from build123d import *

# Parameters (mm, degrees)
SKIZZE1_R                            = 6.1
AUFSATZ_LINEAR_AUSTRAGEN1_DEPTH      = 6
SCHNITT_LINEAR_AUSTRAGEN1_REACH      = 48.187
SCHNITT_LINEAR_AUSTRAGEN1_END_RADIUS = 6.1
SKIZZE2_R                            = 2.2
VERRUNDUNG1_R                        = 6
FASE1_SIZE                           = 0.5


with BuildPart() as part:
    # Skizze1 → Aufsatz-Linear austragen1 (new body)
    with BuildSketch(Plane.XY):
        with BuildLine():
            Line((-3, -12.6), (3, -12.6))
            ThreePointArc((3, -12.6), (8.815176648, -9.489608035), (12.34506932, -3.919089625))
            Line((12.34506932, -3.919089625), (0, 31.5))
            Line((0, 31.5), (-12.34506932, -3.919089625))
            ThreePointArc((-12.34506932, -3.919089625), (-8.815176648, -9.489608035), (-3, -12.6))
        make_face()
        Circle(SKIZZE1_R, mode=Mode.SUBTRACT)
    extrude(amount=AUFSATZ_LINEAR_AUSTRAGEN1_DEPTH)

    # Schnitt-Linear austragen1: up to this cylinder (the profile starts outside it)
    schnitt_linear_austragen1_end = Plane(origin=(0, 0, 3), z_dir=(0, 0, -1)) * Cylinder(SCHNITT_LINEAR_AUSTRAGEN1_END_RADIUS, 109.574, mode=Mode.PRIVATE)
    # Skizze2 → Schnitt-Linear austragen1 (cut, up to the surface)
    with BuildSketch(Plane.XZ.offset(12.6), mode=Mode.PRIVATE) as schnitt_linear_austragen1_sk1:
        with Locations(Location((0, 3, 0), (0, 0, 270))):
            Circle(SKIZZE2_R)
    schnitt_linear_austragen1_tool1 = extrude(schnitt_linear_austragen1_sk1.sketch, amount=-SCHNITT_LINEAR_AUSTRAGEN1_REACH, mode=Mode.PRIVATE) - schnitt_linear_austragen1_end
    add(schnitt_linear_austragen1_tool1.solids().sort_by_distance((0, -12.6, 3))[0], mode=Mode.SUBTRACT)

    # Verrundung1
    verrundung1_edges = [part.edges().sort_by_distance(p)[0] for p in [
        (-12.34506932, -3.919089625, 3),
        (12.34506932, -3.919089625, 3),
    ]]
    fillet(verrundung1_edges, radius=VERRUNDUNG1_R)

    # Fase1
    # the kernel refuses this chamfer: 0.5 mm, written as the material it takes off along each edge
    with BuildSketch(Plane(origin=(0, 0, 6), x_dir=(0.1340527924962947, -0.9909741918051879, 0), z_dir=(-0.9909741918051879, -0.1340527924962947, 0))) as fase1_piece_1:
        Polygon((12.952219887 - FASE1_SIZE, 0), (12.952219887, -FASE1_SIZE), (12.952219887, 0), align=None)
    revolve(axis=Axis((0, 0, 6), (0, 0, 1)), revolution_arc=50.429560745, mode=Mode.SUBTRACT)
    with BuildSketch(Plane(origin=(0, 0, 0), x_dir=(1, 0, 0), z_dir=(0, -1, 0))) as fase1_piece_2:
        Polygon((6.1 + FASE1_SIZE, 0), (6.1, FASE1_SIZE), (6.1, 0), align=None)
    revolve(axis=Axis((0, 0, 0), (0, 0, 1)), mode=Mode.SUBTRACT)
    with BuildSketch(Plane(origin=(0, 0, 6), x_dir=(1, 0, 0), z_dir=(0, -1, 0))) as fase1_piece_3:
        Polygon((6.1 + FASE1_SIZE, 0), (6.1, -FASE1_SIZE), (6.1, 0), align=None)
    revolve(axis=Axis((0, 0, 6), (0, 0, 1)), mode=Mode.SUBTRACT)
    with BuildSketch(Plane(origin=(0.423201699, 32.714202895, 6), x_dir=(0.9439295829747817, -0.32899987713443074, 0.0274958766105856), z_dir=(-0.32912431347143534, -0.9442866017697998, 0)), Plane(origin=(11.570098829, -1.695631129, 6), x_dir=(-0.9439295829747814, -0.32899987713443096, 0.027495876610585616), z_dir=(-0.32912431347143556, 0.9442866017697997, 0))) as fase1_piece_4:
        Polygon((FASE1_SIZE * 0.999621916911, -FASE1_SIZE * 0.0274958766106), (-FASE1_SIZE * 0.0274958766106, -FASE1_SIZE * 0.999621916911), (0, 0), align=None)
    extrude(amount=36.440032041, mode=Mode.SUBTRACT)
    with BuildSketch(Plane(origin=(11.570098829, -1.695631129, 0), x_dir=(-0.9439295829747814, -0.32899987713443096, -0.02749587661058635), z_dir=(-0.32912431347143556, 0.9442866017697997, 0)), Plane(origin=(0.423201699, 32.714202895, 0), x_dir=(0.9439295829747817, -0.32899987713443074, -0.027495876610586334), z_dir=(-0.32912431347143534, -0.9442866017697998, 0))) as fase1_piece_5:
        Polygon((FASE1_SIZE * 0.999621916911, FASE1_SIZE * 0.0274958766106), (-FASE1_SIZE * 0.0274958766106, FASE1_SIZE * 0.999621916911), (0, 0), align=None)
    extrude(amount=36.440032041, mode=Mode.SUBTRACT)
    with BuildSketch(Plane(origin=(0, 0, 0), x_dir=(-0.8492796998321288, -0.5279431706661704, 0), z_dir=(-0.5279431706661704, 0.8492796998321288, 0))) as fase1_piece_6:
        Polygon((12.952219887, FASE1_SIZE), (12.952219887 - FASE1_SIZE, 0), (12.952219887, 0), align=None)
    revolve(axis=Axis((0, 0, 0), (0, 0, 1)), revolution_arc=50.429560745, mode=Mode.SUBTRACT)
    with BuildSketch(Plane(origin=(-5.904379219, -3.67037701, 0), x_dir=(-0.849279699832129, -0.5279431706661702, 0), z_dir=(0.5279431706661702, -0.849279699832129, 0))) as fase1_piece_7:
        Polygon((6 - FASE1_SIZE, 0), (6, -FASE1_SIZE), (6, 0), align=None)
    revolve(axis=Axis((-5.904379219, -3.67037701, 0), (0, 0, -1)), revolution_arc=51.08222172, mode=Mode.SUBTRACT)
    with BuildSketch(Plane(origin=(5.904379219, -3.67037701, 0), x_dir=(0.8492796998321291, -0.5279431706661698, 0), z_dir=(-0.5279431706661698, -0.8492796998321291, 0))) as fase1_piece_8:
        Polygon((6 - FASE1_SIZE, 0), (6, FASE1_SIZE), (6, 0), align=None)
    revolve(axis=Axis((5.904379219, -3.67037701, 0), (0, 0, 1)), revolution_arc=51.08222172, mode=Mode.SUBTRACT)
    with BuildSketch(Plane(origin=(0, 0, 6), x_dir=(-0.8492796998321288, -0.5279431706661704, 0), z_dir=(-0.5279431706661704, 0.8492796998321288, 0))) as fase1_piece_9:
        Polygon((12.952219887, -FASE1_SIZE), (12.952219887 - FASE1_SIZE, 0), (12.952219887, 0), align=None)
    revolve(axis=Axis((0, 0, 6), (0, 0, 1)), revolution_arc=50.429560745, mode=Mode.SUBTRACT)
    with BuildSketch(Plane(origin=(-5.904379219, -3.67037701, 6), x_dir=(-0.849279699832129, -0.5279431706661702, 0), z_dir=(0.5279431706661702, -0.849279699832129, 0))) as fase1_piece_10:
        Polygon((6, FASE1_SIZE), (6 - FASE1_SIZE, 0), (6, 0), align=None)
    revolve(axis=Axis((-5.904379219, -3.67037701, 6), (0, 0, -1)), revolution_arc=51.08222172, mode=Mode.SUBTRACT)
    with BuildSketch(Plane(origin=(5.904379219, -3.67037701, 6), x_dir=(0.8492796998321291, -0.5279431706661698, 0), z_dir=(-0.5279431706661698, -0.8492796998321291, 0))) as fase1_piece_11:
        Polygon((6 - FASE1_SIZE, 0), (6, -FASE1_SIZE), (6, 0), align=None)
    revolve(axis=Axis((5.904379219, -3.67037701, 6), (0, 0, 1)), revolution_arc=51.08222172, mode=Mode.SUBTRACT)
    with BuildSketch(Plane(origin=(0, 0, 0), x_dir=(0.13405279249629465, -0.9909741918051879, 0), z_dir=(-0.9909741918051879, -0.13405279249629465, 0))) as fase1_piece_12:
        Polygon((12.952219887 - FASE1_SIZE, 0), (12.952219887, FASE1_SIZE), (12.952219887, 0), align=None)
    revolve(axis=Axis((0, 0, 0), (0, 0, 1)), revolution_arc=50.429560745, mode=Mode.SUBTRACT)
    with BuildSketch(Plane(origin=(-4.285841494, -12.6, 0), x_dir=(0, 0.9996219169112968, -0.02749587661058644), z_dir=(1, 0, 0)), Plane(origin=(-4.285841494, -12.6, 6), x_dir=(0, -0.027495876610585647, -0.9996219169112968), z_dir=(1, 0, 0))) as fase1_piece_13:
        Polygon((FASE1_SIZE * 0.999621916911, FASE1_SIZE * 0.0274958766106), (-FASE1_SIZE * 0.0274958766106, FASE1_SIZE * 0.999621916911), (0, 0), align=None)
    extrude(amount=8.571682988, mode=Mode.SUBTRACT)


solid = part.part
Could you check a few things on this model? Use its own coordinates, in mm. Give positions to 0.01 mm unless a question says otherwise; leave off trailing zeros. Order: outer loops, then holes, each group sorted by start corner. A loop starts at its lowest first (then second) coordinate and runs counter-clockwise, first axis right, second up. Notation, with made-up numbers: (8.25, 22) -> (47.25, 22) arc R5 cw to (47.25, 29) -> close; hole circle Ø4 at (17, 83). An arc over 180 degrees is marked (long way). Answer in a Markdown table with one row per item. Add a question column.
Item 1: Imagine slicing it at B-B (y = 17). List the corners of the cut face in (x, z) for me, and give its area (3 significant figures).
Item 2: We'd pull the mould along X, two halves only. Please class faces 1 (the flat face through (5, 5, 6)), 2 (the cylindrical face through (-7.627, -10.468, 2.965)), 3 (the cylindrical face through (0.66, -9.19, 0.9)): pulls with the +X half, pulls with the -X half, needs draft (parallel to the pull), parting line crosses it, or undercut.
Item 3: Imagine slicing it at A-A (z = 3). List the corners of the cut face in (x, y) for me, and give its area (3 significant figures).
Item 4: Please list where these lines run through material, in increasing order: probe 1 along Z at (x, y) = (0, -7.75); probe 2 along X at (y, z) = (-8.5, 3); probe 3 along X at (y, z) = (-9, 4.75).
Result:
| question | item | result |
|---|---|---|
| 1 | outline | (-5.05, 0.5) -> (-4.52, 0) -> (4.52, 0) -> (5.05, 0.5) -> (5.05, 5.5) -> (4.52, 6) -> (-4.52, 6) -> (-5.05, 5.5) -> close |
| 1 | area | 60.1 mm2 |
| 2 | face 1 | needs draft |
| 2 | face 2 | pulls with the -X half |
| 2 | face 3 | undercut |
| 3 | outline | (-11.57, -1.7) arc R6 ccw to (-11, -6.84) arc R12.95 ccw to (-3, -12.6) -> (-2.2, -12.6) -> (-2.2, -5.69) arc R6.1 cw (long way) to (2.2, -5.69) -> (2.2, -12.6) -> (3, -12.6) arc R12.95 ccw to (11, -6.84) arc R6 ccw to (11.57, -1.7) -> (0, 31.5) -> close |
| 3 | area | 452 mm2 |
| 4 | probe 1 | 0 to 0.8, 5.2 to 6 |
| 4 | probe 2 | -9.77 to -2.2, 2.2 to 9.77 |
| 4 | probe 3 | -9.31 to -1.33, 1.33 to 9.31 |
